Part model, mm, in its own coordinate system. A direction names the side the tool comes from. Coordinates: 2 decimals unless noted, no trailing zeros. Loops run counter-clockwise (first coordinate to the right, second up) from the corner with the lowest first, then second, coordinate; pieces in that order, holes last. Notation, with made-up numbers: M 3.25,82 L 36.25,82 A11 cw 36.25,93 Z; hole C -15,17 d11. An arc over 180 degrees is marked long. Use a Markdown table: item, result. Add a question column.
1) Band-saw the part on B-B (y = 558.5). List the corners of the cut face in (x, z).
2) Pull direction X, two halves, no side cores. Call faces 4 (the flat face through (306, 523, 6.35)), 5 (the flat face through (450.05, 405.96, 3.13)), 6 (the cylindrical face through (226.51, 584.446, 3.131)): released by +X, released by -X, zero draft, split by the parting line, or undercut.
3) Band-saw the part on A-A (z = 3.5). List the corners of the cut face in (x, y) (1 decimal), plus the area to 3 significant figures.
4) Band-saw the part on C-C (x = 384.5). List the corners of the cut face in (y, z).
5) Wall check: probe 1 along X at (y, z) = (530, 1.25); probe 2 along X at (y, z) = (516.5, 0.5); probe 3 along Y at (x, z) = (455, 5.5). Give the ranges that are in metal, low to high. Write a range as from..to.
6) Pin check, flat tip, straight feed: pin 1 Ø3 at (x, z) = (220, 4.5) entering from -Y. Stop position of the tip, or through.
7) Tool access for faces 1 (the flat face through (306, 523, 0)), 2 (the cylindrical face through (227.708, 542.883, 3.131)), 3 (the flat face through (433.44, 507.99, 3.13)): list every direction of +Z, -Z, +X, -X, +Y, -Y with a clear straight run to the whole face (end or side of a thin tool).
Autodesk Inventor part; units mm, degrees
ref_plane "YZ Plane" through (0, 0, 0) normal (1, 0, 0) x (0, 1, 0)
ref_plane "XZ Plane" through (0, 0, 0) normal (0, 1, 0) x (-1, 0, 0)
ref_plane "XY Plane" through (0, 0, 0) normal (0, 0, 1) x (1, 0, 0)
sketch "Sketch1" plane through (0, 0, 0) normal (0, 0, 1) x (1, 0, 0)
  arc A0 (402.7957, 429.3353) -> (29.7943, 587.9503) centre (0, 0) ccw
  arc A1 (428.864, 457.1212) -> (31.7225, 626.0014) centre (0, 0) ccw
  line L0 (31.7225, 626.0014) -> (32.0439, 632.3433)
  arc A2 (32.0439, 632.3433) -> (13.0183, 633.3074) centre (22.5311, 632.8254) ccw
  line L1 (13.0183, 633.3074) -> (10.4473, 582.5725)
  arc A3 (10.4473, 582.5725) -> (29.4729, 581.6084) centre (19.9601, 582.0905) ccw
  line L2 (29.4729, 581.6084) -> (29.7943, 587.9503)
  line L3 (402.7957, 480.2497) -> (464.9618, 536.5258)
  line L4 (464.9618, 536.5258) -> (496.0072, 536.5258)
  line L5 (496.0072, 536.5258) -> (496.0072, 383.2245)
  line L6 (496.0072, 383.2245) -> (402.7957, 429.3353)
  point P0 (0, 0)
  dimension "d0" = 588.7047
  dimension "d1" = 38.1
  dimension "d2" = 9.525
  dimension "d3" = 50.8
extrude "Extrusion1" add sketch "Sketch1" along normal blind 6.35
properties part number "PLATE,SIDE,RACK,INTAKE"
Entries:
| question | item | result |
|---|---|---|
| 1 | outline | M 186.15,0 L 284.54,0 L 284.54,6.35 L 186.15,6.35 Z |
| 2 | face 4 | zero draft |
| 2 | face 5 | released by -X |
| 2 | face 6 | undercut |
| 3 | outline | M 10.4,582.6 A9.5 ccw 29.5,581.6 L 29.8,588 A588.7 cw 402.8,429.3 L 496,383.2 L 496,536.5 L 465,536.5 L 402.8,480.2 A626.8 ccw 31.7,626 L 32,632.3 A9.5 ccw 13,633.3 Z |
| 3 | area | 27,300 mm2 |
| 4 | outline | M 445.79,0 L 495.02,0 L 495.02,6.35 L 445.79,6.35 Z |
| 5 | probe 1 | 256.27..334.64, 457.75..496.01 |
| 5 | probe 2 | 282.49..355.12, 442.84..496.01 |
| 5 | probe 3 | 403.51..527.51 |
| 6 | pin 1 | y = 545.45 |
| 7 | face 1 | -Z, +X, -X, +Y, -Y |
| 7 | face 2 | +Z, -Z, -Y |
| 7 | face 3 | +Z, -Z, +Y |
